Source: CAD feature listing. Evaluate the final solid. Frame: model axes, mm. A direction names the side the tool comes from. Coordinates: 2 decimals unless noted, no trailing zeros. Loops run counter-clockwise (first coordinate to the right, second up) from the corner with the lowest first, then second, coordinate; pieces in that order, holes last.
Item 1: Pin query (flat end, axial travel): pin 1 Ø2 at (y, z) = (0, 17) entering from -X; pin 2 Ø12 at (x, z) = (71, 2) entering from +Y; pin 3 Ø1 at (x, y) = (40.5, 51.5) entering from -Z. Return the tip coordinate at first contact, or that it passes through.
Item 2: Section query C-C, the plane z = -34. Return the cut outline in (x, y), then the cut area to 3 significant figures.
Item 3: Line query: probe 1 along X at (y, z) = (13.5, -66); probe 2 along X at (y, z) = (48, -48); probe 3 along Z at (x, y) = (43.5, 27). Output: solid intervals per line, ascending.
Item 4: Section query D-D, the plane y = 58. Return the cut outline in (x, z), then the cut area to 3 significant figures.
Item 5: Section query B-B, the plane y = 23. Return the cut outline in (x, z), then the cut area to 3 significant figures.
Item 6: Section query A-A, the plane x = 29.5. State how many separate pieces and enclosed holes the cut face has, then the cut area to 3 significant figures.
Item 7: Reachability of faces 4 (the flat face through (-24, 35, -41.047)), 5 (the flat face through (100, 10, -61)), 6 (the flat face through (44, -3, -31)), 7 (the flat face through (1.161, 1, -83)), 8 (the flat face through (44, 1, 25.572)) from +Z, -Z, +X, -X, +Y, -Y: full face, straight path, thin tool, end or side. Return the list, or none.
Item 8: Pull-direction query (X, two-part tool) for faces 1 (the cylindrical face through (-24.48, 32.99, -76.15)), 2 (the flat face through (45, 1, 20.572)), 3 (the flat face through (50, 70, 11)); classes: +X half, -X half, draft (parallel to the pull), parting line (faces both ways), or undercut.
```python
from build123d import *

# Parameters (mm, degrees)
CORPO_CENTRALE_DEPTH = 70
SCHIZZO13_W          = 18
SCHIZZO13_H          = 12
ON_OFF_DEPTH         = 3
FONDO_START          = 3
FONDO_DEPTH          = 3
MANIGLIA_1_DEPTH     = 10
RACCORDO55_R         = 2.5
RACCORDO56_R         = 2.5
RACCORDO57_R         = 2.5
RACCORDO58_R         = 2.5
RACCORDO62_R         = 2.5
RACCORDO63_R         = 2.5
RACCORDO64_R         = 2.5
RACCORDO65_R         = 2.5
SCHIZZO25_R          = 2.5
ATTACCO_PCB_DEPTH    = 10
CASE_BATTERIA_DEPTH  = 45


with BuildPart() as part:
    # Schizzo2 → Corpo centrale (new body)
    with BuildSketch(Plane(origin=(0, 0, 0), x_dir=(1, 0, 0), z_dir=(0, 1, 0))):
        with BuildLine():
            Line((-22.339499477, 77.047489197), (111.660500523, 77.047489197))
            ThreePointArc((111.660500523, 77.047489197), (113.781820867, 76.168809541), (114.660500523, 74.047489197))
            Line((114.660500523, 74.047489197), (114.660500523, -9.952510803))
            ThreePointArc((114.660500523, -9.952510803), (113.781820867, -12.073831146), (111.660500523, -12.952510803))
            Line((111.660500523, -12.952510803), (-22.339499477, -12.952510803))
            ThreePointArc((-22.339499477, -12.952510803), (-24.460819821, -12.073831146), (-25.339499477, -9.952510803))
            Line((-25.339499477, -9.952510803), (-25.339499477, 74.047489197))
            ThreePointArc((-25.339499477, 74.047489197), (-24.460819821, 76.168809541), (-22.339499477, 77.047489197))
        make_face()
        Polygon((-22.339499477, 71.047489197), (-19.339499477, 71.047489197), (-19.339499477, 74.047489197), (108.660500523, 74.047489197), (108.660500523, 71.047489197), (111.660500523, 71.047489197), (111.660500523, -6.952510803), (108.660500523, -6.952510803), (108.660500523, -9.952510803), (-19.339499477, -9.952510803), (-19.339499477, -6.952510803), (-22.339499477, -6.952510803), align=None, mode=Mode.SUBTRACT)
    extrude(amount=CORPO_CENTRALE_DEPTH)

    # Schizzo13 → On/off (cut)
    with BuildSketch(Plane.ZY.offset(25.339499477)):
        with Locations((-32.047489197, 35)):
            Rectangle(SCHIZZO13_W, SCHIZZO13_H)
    extrude(amount=-ON_OFF_DEPTH, mode=Mode.SUBTRACT)

    # Schizzo18 → Fondo (add)
    with BuildSketch(Plane.XZ.offset(FONDO_START)):
        with BuildLine():
            Line((-25.339499477, 9.952510803), (-25.339499477, -74.047489197))
            ThreePointArc((-25.339499477, -74.047489197), (-24.460819821, -76.168809541), (-22.339499477, -77.047489197))
            Line((-22.339499477, -77.047489197), (111.660500523, -77.047489197))
            ThreePointArc((111.660500523, -77.047489197), (113.781820867, -76.168809541), (114.660500523, -74.047489197))
            Line((114.660500523, -74.047489197), (114.660500523, 9.952510803))
            ThreePointArc((114.660500523, 9.952510803), (113.781820867, 12.073831146), (111.660500523, 12.952510803))
            Line((111.660500523, 12.952510803), (-22.339499477, 12.952510803))
            ThreePointArc((-22.339499477, 12.952510803), (-24.460819821, 12.073831146), (-25.339499477, 9.952510803))
        make_face()
    extrude(amount=-FONDO_DEPTH)

    # Schizzo23 → Maniglia 1 (add)
    with BuildSketch(Plane.XZ.offset(3)):
        with BuildLine():
            Line((1.160500523, 12.952510803), (1.160500523, 23.072411806))
            ThreePointArc((1.160500523, 23.072411806), (1.89273357, 24.840178759), (3.660500523, 25.572411806))
            Line((3.660500523, 25.572411806), (85.660500523, 25.572411806))
            ThreePointArc((85.660500523, 25.572411806), (87.428267476, 24.840178759), (88.160500523, 23.072411806))
            Line((88.160500523, 23.072411806), (88.160500523, 12.952510803))
            Line((88.160500523, 12.952510803), (83.160500523, 12.952510803))
            Line((83.160500523, 12.952510803), (83.160500523, 18.072411806))
            ThreePointArc((83.160500523, 18.072411806), (82.428267476, 19.840178759), (80.660500523, 20.572411806))
            Line((80.660500523, 20.572411806), (8.660500523, 20.572411806))
            ThreePointArc((8.660500523, 20.572411806), (6.89273357, 19.840178759), (6.160500523, 18.072411806))
            Line((6.160500523, 18.072411806), (6.160500523, 12.952510803))
            Line((6.160500523, 12.952510803), (1.160500523, 12.952510803))
        make_face()
    maniglia_1 = extrude(amount=-MANIGLIA_1_DEPTH)

    # Maniglia 2: Maniglia 1 across plane
    add(maniglia_1.mirror(Plane.XY.offset(-32.047489197)))

    # Raccordo55
    raccordo55_edges = [part.edges().sort_by_distance(p)[0] for p in [
        (1.160500523, 7, 18.012461305),
        (1.89273357, 7, 24.840178759),
        (44.660500523, 7, 25.572411806),
        (87.428267476, 7, 24.840178759),
        (88.160500523, 7, 18.012461305),
    ]]
    fillet(raccordo55_edges, radius=RACCORDO55_R)

    # Raccordo56
    raccordo56_edges = [part.edges().sort_by_distance(p)[0] for p in [
        (82.428267476, 7, 19.840178759),
        (83.160500523, 7, 15.512461305),
        (44.660500523, 7, 20.572411806),
        (6.89273357, 7, 19.840178759),
        (6.160500523, 7, 15.512461305),
    ]]
    fillet(raccordo56_edges, radius=RACCORDO56_R - 0.0001)  # a hair under: the kernel refuses the full size

    # Raccordo57
    raccordo57_edges = [part.edges().sort_by_distance(p)[0] for p in [
        (1.160500523, 0.75, 12.952510803),
        (1.89273357, 6.267766953, 12.952510803),
        (6.160500523, 0.75005, 12.952510803),
        (5.428296765, 6.267796242, 12.952510803),
    ]]
    fillet(raccordo57_edges, radius=RACCORDO57_R)

    # Raccordo58
    raccordo58_edges = [part.edges().sort_by_distance(p)[0] for p in [
        (88.160500523, 0.75, 12.952510803),
        (87.428267476, 6.267766953, 12.952510803),
        (83.160500523, 0.75005, 12.952510803),
        (83.892704281, 6.267796242, 12.952510803),
    ]]
    fillet(raccordo58_edges, radius=RACCORDO58_R)

    # Raccordo62
    raccordo62_edges = [part.edges().sort_by_distance(p)[0] for p in [
        (88.160500523, 7, -82.107439699),
        (87.428267476, 7, -88.935157154),
        (44.660500523, 7, -89.667390201),
        (1.89273357, 7, -88.935157154),
        (1.160500523, 7, -82.107439699),
    ]]
    fillet(raccordo62_edges, radius=RACCORDO62_R)

    # Raccordo63
    raccordo63_edges = [part.edges().sort_by_distance(p)[0] for p in [
        (82.428267476, 7, -83.935157154),
        (6.160500523, 7, -79.607439699),
        (6.89273357, 7, -83.935157154),
        (44.660500523, 7, -84.667390201),
        (83.160500523, 7, -79.607439699),
    ]]
    fillet(raccordo63_edges, radius=RACCORDO63_R - 0.0001)  # a hair under: the kernel refuses the full size

    # Raccordo64
    raccordo64_edges = [part.edges().sort_by_distance(p)[0] for p in [
        (88.160500523, 0.75, -77.047489197),
        (87.428267476, 6.267766953, -77.047489197),
        (83.160500523, 0.75005, -77.047489197),
        (83.892704281, 6.267796242, -77.047489197),
    ]]
    fillet(raccordo64_edges, radius=RACCORDO64_R)

    # Raccordo65
    raccordo65_edges = [part.edges().sort_by_distance(p)[0] for p in [
        (1.160500523, 0.75, -77.047489197),
        (1.89273357, 6.267766953, -77.047489197),
        (6.160500523, 0.75005, -77.047489197),
        (5.428296765, 6.267796242, -77.047489197),
    ]]
    fillet(raccordo65_edges, radius=RACCORDO65_R)

    # Schizzo25 → Attacco PCB (add)
    with BuildSketch(Plane(origin=(0, 0, 0), x_dir=(1, 0, 0), z_dir=(0, 1, 0))):
        with Locations(Location((99.660500523, 60.547489197, 0), (0, 0, 90))):
            Circle(SCHIZZO25_R)
        with Locations(Location((102.660500523, 0.547489197, 0), (0, 0, 90))):
            Circle(SCHIZZO25_R)
        with Locations(Location((16.660500523, 3.547489197, 0), (0, 0, 90))):
            Circle(SCHIZZO25_R)
        with Locations(Location((16.660500523, 60.547489197, 0), (0, 0, 90))):
            Circle(SCHIZZO25_R)
    extrude(amount=ATTACCO_PCB_DEPTH)

    # Schizzo26 → Case Batteria (add)
    with BuildSketch(Plane(origin=(0, 0, 0), x_dir=(1, 0, 0), z_dir=(0, 1, 0))):
        Polygon((-13.339499477, 74.047489197), (-15.339499477, 74.047489197), (-15.339499477, 44.047489197), (7.660500523, 44.047489197), (7.660500523, 74.047489197), (5.660500523, 74.047489197), (5.660500523, 46.047489197), (-13.339499477, 46.047489197), align=None)
    extrude(amount=CASE_BATTERIA_DEPTH)


solid = part.part
```
Verdict:
1. pin 1: stops at x = 1.16
1. pin 2: stops at y = 0
1. pin 3: stops at z = -77.05
2. outline: (-25.34, -3) - (114.66, -3) - (114.66, 70) - (111.66, 70) - (111.66, 0) - (-22.34, 0) - (-22.34, 29) - (-25.34, 29) - close; (-25.34, 41) - (-22.34, 41) - (-22.34, 70) - (-25.34, 70) - close
2. area: 804 mm2
3. probe 1: x = -25.34 to -22.34, -15.34 to -13.34, 5.66 to 7.66, 111.66 to 114.66
3. probe 2: x = -25.34 to -22.34, 111.66 to 114.66
3. probe 3: z = -77.05 to -74.05, 9.95 to 12.95
4. outline: (-25.34, -74.05) arc R3 ccw to (-22.34, -77.05) - (111.66, -77.05) arc R3 ccw to (114.66, -74.05) - (114.66, 9.95) arc R3 ccw to (111.66, 12.95) - (-22.34, 12.95) arc R3 ccw to (-25.34, 9.95) - close; hole (-22.34, -71.05) - (-19.34, -71.05) - (-19.34, -74.05) - (108.66, -74.05) - (108.66, -71.05) - (111.66, -71.05) - (111.66, 6.95) - (108.66, 6.95) - (108.66, 9.95) - (-19.34, 9.95) - (-19.34, 6.95) - (-22.34, 6.95) - close
4. area: 1,370 mm2
5. outline: (-25.34, -74.05) arc R3 ccw to (-22.34, -77.05) - (111.66, -77.05) arc R3 ccw to (114.66, -74.05) - (114.66, 9.95) arc R3 ccw to (111.66, 12.95) - (-22.34, 12.95) arc R3 ccw to (-25.34, 9.95) - close; hole (-22.34, -71.05) - (-19.34, -71.05) - (-19.34, -74.05) - (-15.34, -74.05) - (-15.34, -44.05) - (7.66, -44.05) - (7.66, -74.05) - (108.66, -74.05) - (108.66, -71.05) - (111.66, -71.05) - (111.66, 6.95) - (108.66, 6.95) - (108.66, 9.95) - (-19.34, 9.95) - (-19.34, 6.95) - (-22.34, 6.95) - close; hole (-13.34, -74.05) - (5.66, -74.05) - (5.66, -46.05) - (-13.34, -46.05) - close
5. area: 1,530 mm2
6. separate pieces: 3
6. enclosed holes: 0
6. area: 785 mm2
7. face 4: -X
7. face 5: +Y
7. face 6: +Z, -Z, +X, -X, -Y
7. face 7: -Z, -X, +Y, -Y
7. face 8: +Z, +X, -X, +Y, -Y
8. face 1: -X half
8. face 2: undercut
8. face 3: draft
